Source: CAD feature listing. Evaluate the final solid. Frame: model axes, mm. A direction names the side the tool comes from. Give positions to 0.01 mm unless a question says otherwise; leave off trailing zeros. Loops run counter-clockwise (first coordinate to the right, second up) from the corner with the lowest first, then second, coordinate; pieces in that order, holes last.
```python
from build123d import *

# Parameters (mm, degrees)
F0_R           = 25.4
F0_R_2         = 12.7
F1_DEPTH       = 76.2
F4_DEPTH       = 25.4
F4_DEPTH_BACK  = 12.7
F5_R           = 12.7
F6_DEPTH       = 76.201
F7_W           = 25.4
F7_H           = 12.7
F8_DEPTH       = 76.201
F10_DEPTH      = 25.4
F10_DEPTH_BACK = 25.4


with BuildPart() as f1:
    # F0 (on Right) → F1 (new body)
    with BuildSketch(Plane.YZ):
        Circle(F0_R)
        Circle(F0_R_2, mode=Mode.SUBTRACT)
    extrude(amount=F1_DEPTH)

    # F3 (on Front) → F4 (join, two sides)
    with BuildSketch(Plane.XZ) as f4_sk:
        Polygon((0, 50.8), (0, 0), (38.1, 0), align=None)
    extrude(amount=-F4_DEPTH)
    extrude(f4_sk.sketch, amount=F4_DEPTH_BACK)

    # F5 (on face) → F6 (cut, through all)
    with BuildSketch(Plane.YZ.offset(76.2)):
        Circle(F5_R)
    extrude(amount=-F6_DEPTH, mode=Mode.SUBTRACT)

    # F7 (on face) → F8 (cut, through all)
    with BuildSketch(Plane.YZ):
        with Locations((0, 44.45)):
            Rectangle(F7_W, F7_H)
    extrude(amount=F8_DEPTH, mode=Mode.SUBTRACT)

    # F9 (on Front) → F10 (cut, two sides)
    with BuildSketch(Plane.XZ) as f10_sk:
        Polygon((76.2, 25.4035045986), (50.8, 25.4035045986), (50.8, -9.5214954014), (63.5, -9.5214954014), (63.5, 9.5285045986), (76.2, 9.5285045986), align=None)
    extrude(amount=-F10_DEPTH, mode=Mode.SUBTRACT)
    extrude(f10_sk.sketch, amount=F10_DEPTH_BACK, mode=Mode.SUBTRACT)


solid = f1.part
```
(1) Section C-C, the plane z = 23. Return the cut outline in (x, y).
A:
outline: (0, -12.7) - (20.85, -12.7) - (20.85, -10.78) - (50.8, -10.78) - (50.8, 10.78) - (20.85, 10.78) - (20.85, 25.4) - (0, 25.4) - close
(2) Section D-D, the plane y = 15.5. Return the cut outline in (x, z).
A:
outline: (0, -20.12) - (76.2, -20.12) - (76.2, 9.53) - (63.5, 9.53) - (63.5, -9.52) - (50.8, -9.52) - (50.8, 20.12) - (23.01, 20.12) - (0, 50.8) - close
(3) Reachability of faces 4 (the flat face through (63.5, 19, 0)), 5 (the flat face through (70, 16, 9.529)), 6 (the flat face through (76.2, 5, -12)), 7 (the flat face through (5, 0, 38.1)), 8 (the flat face through (10, 25.4, 14)) from +Z, -Z, +X, -X, +Y, -Y: full face, straight path, thin tool, end or side. Return the list, or none.
A:
face 4: +Z, +Y, -Y
face 5: +Z, +X, +Y, -Y
face 6: +Z, -Z, +X, +Y, -Y
face 7: +Z, +X, -X, -Y
face 8: +Z, -Z, +X, -X, +Y
(4) Ray query, line 1 along Y through (x, z) = (46.5, 0); line 2 along X through (y, z) = (18, 6). Return the intervals inside material, ascending.
A:
line 1: y = -25.4 to -12.7, 12.7 to 25.4
line 2: x = 0 to 50.8, 63.5 to 76.2
(5) Section A-A, the plane y = 0. Return the cut outline in (x, z) (3 decimals), then the cut area to 3 significant figures.
A:
outline: (0, -25.4) - (76.2, -25.4) - (76.2, -12.7) - (0, -12.7) - close; (0, 12.7) - (50.8, 12.7) - (50.8, 25.4) - (19.05, 25.4) - (9.525, 38.1) - (0, 38.1) - close
area: 1,790 mm2
(6) Mould query, pull axis X, two halves, no side actions, for faces 1 (the flat face through (15.083, 10.85, 30.689)), 2 (the flat face through (50.8, 5, 12)), 3 (the flat face through (8, -12.7, 28)). Classes: pulls with the +X half, pulls with the -X half, needs draft (parallel to the pull), parting line crosses it, or undercut.
A:
face 1: pulls with the +X half
face 2: undercut
face 3: needs draft
(7) First-contact query: pin 1 (5 mm diameter, centred on x = 48, y = 4, fed in from +Z); pin 2 (5 mm diameter, centred on x = 38.5, z = -2.5, fed in from +Y); pin 3 (8 mm diameter, centred on x = 13.5, z = 32.5, fed in from -Y); pin 4 (6.5 mm diameter, centred on x = 70.5, y = 15, fed in from +Z). Flat tips, straight axial feed; report the tip coordinate or a pass-through.
A:
pin 1: stops at z = 25.36
pin 2: stops at y = 25.4
pin 3: stops at y = -12.7
pin 4: stops at z = 9.53
(8) Section B-B, the plane y = 10. Return the cut outline in (x, z) (1 decimal).
A:
outline: (0, -23.3) - (76.2, -23.3) - (76.2, -7.8) - (63.5, -7.8) - (63.5, -9.5) - (50.8, -9.5) - (50.8, -7.8) - (0, -7.8) - close; (0, 7.8) - (50.8, 7.8) - (50.8, 23.3) - (20.6, 23.3) - (9.5, 38.1) - (0, 38.1) - close; (63.5, 7.8) - (76.2, 7.8) - (76.2, 9.5) - (63.5, 9.5) - close
